Check sheet for the modelled part. Datum: model origin and axes. Units: mm. Round coordinates to 2 decimals unless told otherwise and drop trailing zeros. Loops run counter-clockwise (first coordinate to the right, second up) from the corner with the lowest first, then second, coordinate; pieces in that order, holes last. Notation, with made-up numbers: (36.5, 10.25) - (48.5, 10.25) arc R36 cw to (48.5, 49.25) - close; hole circle Ø7 at (26, 31). An arc over 180 degrees is marked (long way). Put each result on its own line as item: value. Start each with the question number.
Item 1: Section check B-B, the plane z = 19.05. Record the cut outline in (x, y).
Item 2: Material ranges on line 1 along Z through (x, y) = (6.25, 10); line 2 along X through (y, z) = (5.5, 19.05); line 3 along Z through (x, y) = (5.25, 3.5), recorded low to high.
Item 3: Section check D-D, the plane x = 1. Record the cut outline in (y, z).
Item 4: Section check C-C, the plane y = 4.5. Record the cut outline in (x, z), and give its area (3 significant figures).
Item 5: Section check A-A, the plane x = 6.35. Give the number of separate pieces and of enclosed holes in the cut face, and give its area (3 significant figures).
Item 6: Gauge pin test, flat ends, axial feed: pin 1 Ø1.4 at (x, z) = (6.5, -32.5) entering from +Y; pin 2 Ø4 at (x, z) = (7.5, 33) entering from +Y; pin 3 Ø5 at (x, z) = (6.5, -19) entering from +Y. Record the tip position at first contact, or that the pin passes through.
from build123d import *

# Parameters (mm, degrees)
BOSS_EXTRUDE1_DEPTH = 12.7
SKETCH2_R           = 2.286
CUT_EXTRUDE1_DEPTH  = 12.7
FILLET1_R           = 1.27


with BuildPart() as part:
    # Sketch1 → Boss-Extrude1 (new body)
    with BuildSketch(Plane(origin=(0, 0, 0), x_dir=(0, 0, -1), z_dir=(1, 0, 0))):
        Polygon((42.418, 0), (-42.418, 0), (-42.418, 12.7), (-36.068, 12.7), (-36.068, 6.35), (-28.702, 6.35), (-28.702, 12.7), (28.702, 12.7), (28.702, 6.35), (36.068, 6.35), (36.068, 12.7), (42.418, 12.7), align=None)
    extrude(amount=BOSS_EXTRUDE1_DEPTH)

    # Sketch2 → Cut-Extrude1 (cut)
    with BuildSketch(Plane(origin=(0, 12.7, 0), x_dir=(1, 0, 0), z_dir=(0, 1, 0))):
        with Locations(Location((6.35, -19.05, 0), (0, 0, 270))):
            Circle(SKETCH2_R)
        with Locations(Location((6.35, 19.05, 0), (0, 0, 270))):
            Circle(SKETCH2_R)
    extrude(amount=-CUT_EXTRUDE1_DEPTH, mode=Mode.SUBTRACT)

    # Fillet1
    fillet1_edges = [part.edges().sort_by_distance(p)[0] for p in [
        (6.35, 12.7, 42.418),
        (6.35, 12.7, 36.068),
        (6.35, 6.35, 36.068),
        (6.35, 6.35, 28.702),
        (6.35, 12.7, 28.702),
        (6.35, 12.7, -28.702),
        (6.35, 6.35, -28.702),
        (6.35, 6.35, -36.068),
        (6.35, 12.7, -36.068),
        (6.35, 12.7, -42.418),
        (6.35, 0, -42.418),
        (6.35, 0, 42.418),
    ]]
    fillet(fillet1_edges, radius=FILLET1_R)


solid = part.part
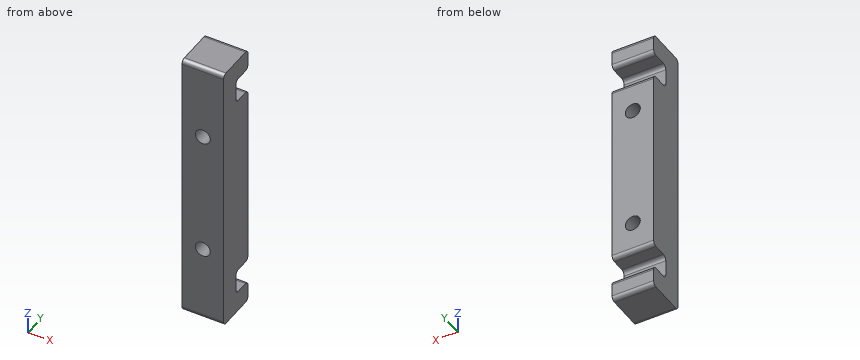
Check result:
1. outline: (0, 0) - (4.06, 0) - (4.06, 12.7) - (0, 12.7) - close; (8.64, 0) - (12.7, 0) - (12.7, 12.7) - (8.64, 12.7) - close
2. line 1: -42.42 to -36.07, -28.7 to -21.33, -16.77 to 16.77, 21.33 to 28.7, 36.07 to 42.42
2. line 2: 0 to 4.06, 8.64 to 12.7
2. line 3: -42.42 to -21.05, -17.05 to 17.05, 21.05 to 42.42
3. outline: (0, -41.15) arc R1.27 ccw to (1.27, -42.42) - (11.43, -42.42) arc R1.27 ccw to (12.7, -41.15) - (12.7, -37.34) arc R1.27 ccw to (11.43, -36.07) - (7.62, -36.07) arc R1.27 cw to (6.35, -34.8) - (6.35, -29.97) arc R1.27 cw to (7.62, -28.7) - (11.43, -28.7) arc R1.27 ccw to (12.7, -27.43) - (12.7, 27.43) arc R1.27 ccw to (11.43, 28.7) - (7.62, 28.7) arc R1.27 cw to (6.35, 29.97) - (6.35, 34.8) arc R1.27 cw to (7.62, 36.07) - (11.43, 36.07) arc R1.27 ccw to (12.7, 37.34) - (12.7, 41.15) arc R1.27 ccw to (11.43, 42.42) - (1.27, 42.42) arc R1.27 ccw to (0, 41.15) - close
4. outline: (0, -42.42) - (12.7, -42.42) - (12.7, 42.42) - (0, 42.42) - close; hole circle Ø4.57 at (6.35, -19.05); hole circle Ø4.57 at (6.35, 19.05)
4. area: 1,040 mm²
5. separate pieces: 3
5. enclosed holes: 0
5. area: 866 mm²
6. pin 1: y = 6.35
6. pin 2: y = 6.37
6. pin 3: y = 12.7
